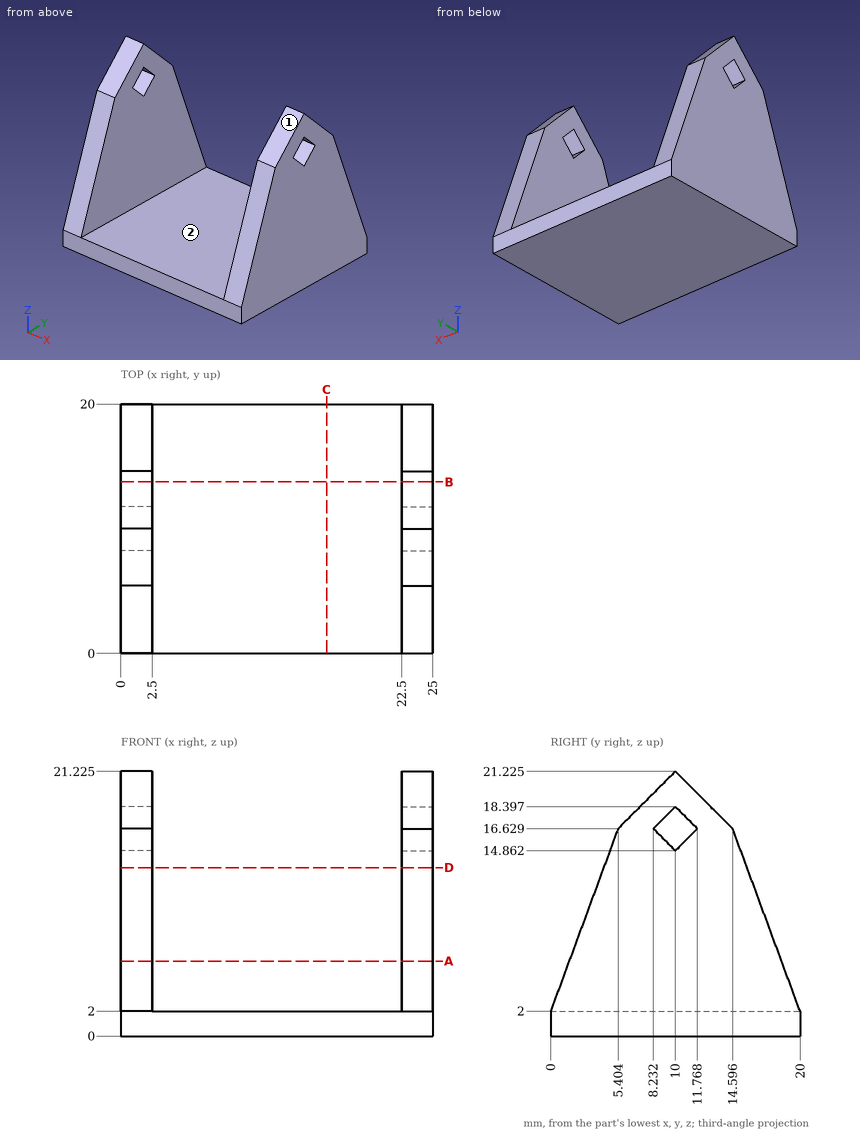
Geometry check sheet. Reference: drawing and pictorial views, mm from the part's lowest x, y, z. A direction names the side the tool comes from. Coordinates: 2 decimals unless noted, no trailing zeros. Order: outer loops, then holes, each group sorted by start corner. A loop starts at its lowest first (then second) coordinate and runs counter-clockwise, first axis right, second up. Notation, with made-up numbers: (75, 19) -> (131, 19) arc R20 ccw to (131, 32) -> close; hole circle Ø9 at (22, 7). An arc over 180 degrees is marked (long way). Use CSV: the item, a comma, the result in double quotes. Start each with the question number.
Q1. Section check D-D, the plane z = 13.5. Record the cut outline in (x, y).
Q2. Thickness scan on line 1 along X through (y, z) = (4.5, 3.5); line 2 along Z through (x, y) = (20.5, 10.75); line 3 along Y through (x, z) = (23.5, 2.75). Record the ranges inside material, lowest first.
Q3. Section check B-B, the plane y = 13.75. Record the cut outline in (x, z) (1 decimal).
Q4. Tool access check on the marked faces 1 and 2. Record the directions out of +Z, -Z, +X, -X, +Y, -Y that give a thin tool (end or side, any length) a straight path to the whole face; none if there is none.
Q5. Section check C-C, the plane x = 16.5. Record the cut outline in (y, z).
Q6. Depth check by flat-ended pin: P1, Ø1, axis at x = 10, y = 11.5, coming from the +Z side; P2, Ø2, axis at x = 18, z = 3.5, coming from the -Y side. Enter the tip coordinate at first touch or a pass-through.
Q7. Section check A-A, the plane z = 6. Record the cut outline in (x, y).
Returned:
1,outline,"(0, 4.25) -> (2.5, 4.25) -> (2.5, 15.75) -> (0, 15.75) -> close; (22.5, 4.25) -> (25, 4.25) -> (25, 15.75) -> (22.5, 15.75) -> close"
2,line 1,"x = 0 to 2.5, 22.5 to 25"
2,line 2,"z = 0 to 2"
2,line 3,"y = 0.28 to 19.72"
3,outline,"(0, 0) -> (25, 0) -> (25, 17.5) -> (22.5, 17.5) -> (22.5, 2) -> (2.5, 2) -> (2.5, 17.5) -> (0, 17.5) -> close"
4,face 1,"+Z, +X, -X, -Y"
4,face 2,"+Z, +Y, -Y"
5,outline,"(0, 0) -> (20, 0) -> (20, 2) -> (0, 2) -> close"
6,P1,"stops at z = 2"
6,P2,"passes through"
7,outline,"(0, 1.48) -> (2.5, 1.48) -> (2.5, 18.52) -> (0, 18.52) -> close; (22.5, 1.48) -> (25, 1.48) -> (25, 18.52) -> (22.5, 18.52) -> close"
